from build123d import *

# Parameters (mm, degrees)
SKETCH1_R           = 1.2065
SKETCH1_R_2         = 1.4605
SKETCH1_W           = 6.35
SKETCH1_H           = 2.9972
BOSS_EXTRUDE1_DEPTH = 2.9972
FILLET1_R           = 3.175
FILLET2_START       = -1
FILLET2_DEPTH       = 5
FILLET2_2_DEPTH     = 2.9972


with BuildPart() as part:
    # Sketch1 → Boss-Extrude1 (new body)
    with BuildSketch(Plane(origin=(0, 0, 0), x_dir=(1, 0, 0), z_dir=(0, 1, 0))):
        Polygon((-11.43, -11.43), (-11.43, -19.05), (-6.096, -19.05), (-6.096, -37.465), (0, -37.465), (6.096, -37.465), (6.096, -19.05), (11.43, -19.05), (11.43, -11.43), (11.43, 11.43), (-11.43, 11.43), align=None)
        with Locations(Location((-7.747, 0, 0), (0, 0, 90))):
            Circle(SKETCH1_R, mode=Mode.SUBTRACT)
        with Locations(Location((7.747, 0, 0), (0, 0, 90))):
            Circle(SKETCH1_R, mode=Mode.SUBTRACT)
        with Locations(Location((0, -24.13, 0), (0, 0, 90))):
            Circle(SKETCH1_R_2, mode=Mode.SUBTRACT)
        with Locations(Location((0, -31.369, 0), (0, 0, 90))):
            Circle(SKETCH1_R_2, mode=Mode.SUBTRACT)
        with Locations((6.35, 8.0264)):
            Rectangle(SKETCH1_W, SKETCH1_H, mode=Mode.SUBTRACT)
        with Locations((-6.35, -8.0264)):
            Rectangle(SKETCH1_W, SKETCH1_H, mode=Mode.SUBTRACT)
        with Locations((6.35, -8.0264)):
            Rectangle(SKETCH1_W, SKETCH1_H, mode=Mode.SUBTRACT)
        with Locations((-6.35, 8.0264)):
            Rectangle(SKETCH1_W, SKETCH1_H, mode=Mode.SUBTRACT)
    extrude(amount=BOSS_EXTRUDE1_DEPTH)

    # Fillet1
    fillet1_edges = [part.edges().sort_by_distance(p)[0] for p in [
        (-6.096, 1.4986, 37.465),
        (-11.43, 1.4986, -11.43),
        (11.43, 1.4986, -11.43),
        (6.096, 1.4986, 37.465),
    ]]
    fillet(fillet1_edges, radius=FILLET1_R)

    # Fillet2: read off the stored shape, not the designer's step
    # Fillet2 outline → Fillet2 (cut)
    with BuildSketch(Plane(origin=(0, 0, 0), x_dir=(1, 0, 0), z_dir=(0, 1, 0)).offset(FILLET2_START)):
        with BuildLine():
            ThreePointArc((11.43, -16.383), (10.648853785, -18.268853785), (8.763, -19.05))
            Line((8.763, -19.05), (11.43, -19.05))
            Line((11.43, -19.05), (11.43, -16.383))
        make_face()
        with BuildLine():
            Line((-11.43, -19.05), (-8.763, -19.05))
            ThreePointArc((-8.763, -19.05), (-10.648853785, -18.268853785), (-11.43, -16.383))
            Line((-11.43, -16.383), (-11.43, -19.05))
        make_face()
    extrude(amount=FILLET2_DEPTH, mode=Mode.SUBTRACT)

    # Fillet2 2 outline → Fillet2 2 (add)
    with BuildSketch(Plane(origin=(0, 0, 0), x_dir=(1, 0, 0), z_dir=(0, 1, 0))):
        with BuildLine():
            ThreePointArc((6.096, -21.717), (6.877146215, -19.831146215), (8.763, -19.05))
            Line((8.763, -19.05), (6.096, -19.05))
            Line((6.096, -19.05), (6.096, -21.717))
        make_face()
        with BuildLine():
            Line((-6.096, -19.05), (-8.763, -19.05))
            ThreePointArc((-8.763, -19.05), (-6.877146215, -19.831146215), (-6.096, -21.717))
            Line((-6.096, -21.717), (-6.096, -19.05))
        make_face()
    extrude(amount=FILLET2_2_DEPTH)


solid = part.part
Design review of the part built by this model. Coordinates are the model's own, in mm. A direction names the side the tool comes from. Round coordinates to 2 decimals unless told otherwise and drop trailing zeros. Loops run counter-clockwise (first coordinate to the right, second up) from the corner with the lowest first, then second, coordinate; pieces in that order, holes last. Notation, with made-up numbers: (-28.75, 43) - (30.25, 43) arc R26 ccw to (30.25, 62) - close; hole circle Ø6 at (11.5, 43.5). An arc over 180 degrees is marked (long way). One line per question, with ' | ' between items.
1. Clearance check with flat-ended pins moving along their axes: P1, Ø0.9, axis at x = -5.5, y = 1.5, coming from the +Z side; P2, Ø1.5, axis at x = 7.5, y = 1, coming from the +Z side. State where each tip first meets the part, or that it passes through.
Results are:
P1: stops at z = 36.65 | P2: stops at z = 19.97
2. For faces 5 (the face through (6.096, 1, 28)), 6 (the face through (-10.5, 1.5, -10.5)), 7 (the face through (-9.525, 1, -8)), list the 3-axis set-ups (+Z, -Z, +X, -X, +Y, -Y) from which the entire face can be reached by the end or side of a thin tool; tool diameter is ignored.
Results are:
face 5: +Z, +X, +Y, -Y | face 6: -Z, -X, +Y, -Y | face 7: +Y, -Y
3. For L1, parallel to X at y = 0.7, z = 0; L2, parallel to X at y = 0.8, z = 8 (3 decimals); L3, parallel to X at y = 1.1, z = 24.13, list the stretches that pass through material, from the lowest coordinate up. Write a range as [from, to].
Results are:
L1: x = [-11.43, -8.95], [-6.54, 6.54], [8.95, 11.43] | L2: x = [-11.43, -9.525], [-3.175, 3.175], [9.525, 11.43] | L3: x = [-6.1, -1.46], [1.46, 6.1]
4. We need section C-C, the plane z = 0. State the section outline as (x, y) points, and give its area (3 significant figures).
Results are:
outline: (-11.43, 0) - (-8.95, 0) - (-8.95, 3) - (-11.43, 3) - close; (-6.54, 0) - (6.54, 0) - (6.54, 3) - (-6.54, 3) - close; (8.95, 0) - (11.43, 0) - (11.43, 3) - (8.95, 3) - close | area: 54.1 mm²
5. We need section A-A, the plane z = 24.13. State the section outline as (x, y) points.
Results are:
outline: (-6.1, 0) - (-1.46, 0) - (-1.46, 3) - (-6.1, 3) - close; (1.46, 0) - (6.1, 0) - (6.1, 3) - (1.46, 3) - close
6. Draft analysis for pull direction Z (two halves, no side actions). For faces 1 (the face through (-3.175, 1, 8)), 2 (the face through (0, 1, -11.43)), 3 (the face through (0, 0, 13)), 4 (the face through (-8.764, 1.478, -0.649)), state which applies: released by +Z, released by -Z, zero draft, split by the parting line, or undercut.
Results are:
face 1: undercut | face 2: released by -Z | face 3: zero draft | face 4: undercut
7. We need section D-D, the plane x = -7. State the section outline as (y, z) points (3 decimals).
Results are:
outline: (0, -11.43) - (2.997, -11.43) - (2.997, -9.525) - (0, -9.525) - close; (0, -6.528) - (2.997, -6.528) - (2.997, -0.947) - (0, -0.947) - close; (0, 0.947) - (2.997, 0.947) - (2.997, 6.528) - (0, 6.528) - close; (0, 9.525) - (2.997, 9.525) - (2.997, 19.716) - (0, 19.716) - close
8. We need section B-B, the plane x = 0. State the section outline as (y, z) points (1 decimal).
Results are:
outline: (0, -11.4) - (3, -11.4) - (3, 22.7) - (0, 22.7) - close; (0, 25.6) - (3, 25.6) - (3, 29.9) - (0, 29.9) - close; (0, 32.8) - (3, 32.8) - (3, 37.5) - (0, 37.5) - close
